from build123d import *

# Parameters (mm, degrees)
F0_W     = 252
F0_H     = 252
F1_DEPTH = 30
F3_DEPTH = 20
F5_D     = 8.5


with BuildPart() as f1:
    # F0 (on Front) → F1 (new body)
    with BuildSketch(Plane.XZ):
        with Locations((126, 126)):
            Rectangle(F0_W, F0_H)
    extrude(amount=F1_DEPTH)

    # F2 (on face) → F3 (cut)
    with BuildSketch(Plane.XZ.offset(30)):
        with BuildLine():
            Line((7, 26), (0, 26))
            Line((0, 26), (0, 12))
            Line((0, 12), (7, 12))
            ThreePointArc((7, 12), (14, 19), (7, 26))
        make_face()
        with BuildLine():
            Line((245, 12), (252, 12))
            Line((252, 12), (252, 26))
            Line((252, 26), (245, 26))
            ThreePointArc((245, 26), (238, 19), (245, 12))
        make_face()
        with BuildLine():
            Line((252, 226), (252, 240))
            Line((252, 240), (245, 240))
            ThreePointArc((245, 240), (238, 233), (245, 226))
            Line((245, 226), (252, 226))
        make_face()
        with BuildLine():
            Line((0, 233), (0, 226))
            Line((0, 226), (7, 226))
            ThreePointArc((7, 226), (14, 233), (7, 240))
            Line((7, 240), (0, 240))
            Line((0, 240), (0, 233))
        make_face()
    extrude(amount=-F3_DEPTH, mode=Mode.SUBTRACT)

    # F5 (through all)
    with Locations(Plane.XZ.offset(10)):
        with Locations((7, 233), (245, 233), (245, 19), (7, 19)):
            Hole(F5_D / 2)


solid = f1.part
Verification items for the finished model (mm, model axes). A direction names the side the tool comes from. Coordinates: 2 decimals unless noted, no trailing zeros. Order: outer loops, then holes, each group sorted by start corner. A loop starts at its lowest first (then second) coordinate and runs counter-clockwise, first axis right, second up. Notation, with made-up numbers: M 80.25,57.5 L 98.25,57.5 A23 cw 98.25,66.5 Z; hole C 6.5,-13 d9. An arc over 180 degrees is marked long. One line per item, written item: value. Start each with the question number.
Item 1: Access from +Z, -Z, +X, -X, +Y, -Y to the whole of each face (thin tool, end or side, straight path). Record for faces 4 (the cylindrical face through (238, -20, 19)), 5 (the flat face through (3, -20, 12)), 6 (the flat face through (124, 0, 128)).
Item 2: Thickness scan on probe 1 along Z at (x, y) = (7, -7); probe 2 along X at (y, z) = (-4.5, 22). Record the ranges inside material, lowest first.
Item 3: Depth check by flat-ended pin: P1, Ø7.5, axis at x = 249, y = -19.5, coming from the -Z side; P2, Ø7, axis at x = 246.5, z = 236, coming from the -Y side. Enter the tip coordinate at first touch or a pass-through.
Item 4: Mould release check, pull along Z, two halves, no side actions. Record for faces 1 (the flat face through (4, -20, 240)), 2 (the flat face through (124, -15, 0)), 3 (the flat face through (124, -30, 128)): pulls with the +Z half, pulls with the -Z half, needs draft (parallel to the pull), parting line crosses it, or undercut.
Item 5: Sectioned sample at A-A on z = 19. Record the cut outline in (x, y).
Calculated:
1. face 4: +X, -Y
1. face 5: -X, -Y
1. face 6: +Z, -Z, +X, -X, +Y
2. probe 1: 0 to 14.75, 23.25 to 228.75, 237.25 to 252
2. probe 2: 0 to 3.99, 10.01 to 241.99, 248.01 to 252
3. P1: z = 0
3. P2: y = -10
4. face 1: undercut
4. face 2: pulls with the -Z half
4. face 3: needs draft
5. outline: M 0,-10 L 2.75,-10 L 2.75,0 L 0,0 Z; M 11.25,-10 L 14,-10 L 14,-30 L 238,-30 L 238,-10 L 240.75,-10 L 240.75,0 L 11.25,0 Z; M 249.25,-10 L 252,-10 L 252,0 L 249.25,0 Z
